```python
from build123d import *

# Parameters (mm, degrees)
SKETCH1_W               = 249.6
SKETCH1_H               = 340.9
SKETCH1_R               = 2.1
SKETCH1_R_2             = 2.5
SKETCH1_R_3             = 1.59
SKETCH1_R_4             = 12.5
SKETCH1_W_2             = 33
SKETCH1_H_2             = 90
BOSS_EXTRUDE1_DEPTH     = 5
CUT_EXTRUDE3_DEPTH      = 193
CUT_EXTRUDE3_DEPTH_BACK = 193
CUT_EXTRUDE6_DEPTH      = 6
SKETCH8_R               = 2
SKETCH8_R_2             = 2.1
SKETCH8_R_3             = 2.058578644
SKETCH8_R_4             = 4
SKETCH8_R_5             = 4.3
CUT_EXTRUDE7_DEPTH      = 6
SKETCH9_R               = 12.5
SKETCH9_R_2             = 2.1
CUT_EXTRUDE8_DEPTH      = 6


with BuildPart() as part:
    # Sketch1 → Boss-Extrude1 (new body)
    with BuildSketch(Plane.XY):
        with Locations((124.8, -170.45)):
            Rectangle(SKETCH1_W, SKETCH1_H)
        with Locations((104.3, -14)):
            Circle(SKETCH1_R, mode=Mode.SUBTRACT)
        with Locations((245.6, -26.5)):
            Circle(SKETCH1_R_2, mode=Mode.SUBTRACT)
        with Locations((245.6, -77.5)):
            Circle(SKETCH1_R_2, mode=Mode.SUBTRACT)
        with Locations((145.3, -14)):
            Circle(SKETCH1_R, mode=Mode.SUBTRACT)
        with Locations((179.16, -36.375)):
            Circle(SKETCH1_R_3, mode=Mode.SUBTRACT)
        with Locations((179.16, -67.625)):
            Circle(SKETCH1_R_3, mode=Mode.SUBTRACT)
        with Locations((124.8, -14)):
            Circle(SKETCH1_R_4, mode=Mode.SUBTRACT)
        with Locations((141.06, -36.375)):
            Circle(SKETCH1_R_3, mode=Mode.SUBTRACT)
        with Locations((153.76, -36.375)):
            Circle(SKETCH1_R_3, mode=Mode.SUBTRACT)
        with Locations((166.46, -36.375)):
            Circle(SKETCH1_R_3, mode=Mode.SUBTRACT)
        with Locations((141.06, -67.625)):
            Circle(SKETCH1_R_3, mode=Mode.SUBTRACT)
        with Locations((153.76, -67.625)):
            Circle(SKETCH1_R_3, mode=Mode.SUBTRACT)
        with Locations((166.46, -67.625)):
            Circle(SKETCH1_R_3, mode=Mode.SUBTRACT)
        with Locations((83.14, -67.625)):
            Circle(SKETCH1_R_3, mode=Mode.SUBTRACT)
        with Locations((95.84, -67.625)):
            Circle(SKETCH1_R_3, mode=Mode.SUBTRACT)
        with Locations((108.54, -67.625)):
            Circle(SKETCH1_R_3, mode=Mode.SUBTRACT)
        with Locations((83.14, -36.375)):
            Circle(SKETCH1_R_3, mode=Mode.SUBTRACT)
        with Locations((95.84, -36.375)):
            Circle(SKETCH1_R_3, mode=Mode.SUBTRACT)
        with Locations((108.54, -36.375)):
            Circle(SKETCH1_R_3, mode=Mode.SUBTRACT)
        with Locations((70.44, -67.625)):
            Circle(SKETCH1_R_3, mode=Mode.SUBTRACT)
        with Locations((70.44, -36.375)):
            Circle(SKETCH1_R_3, mode=Mode.SUBTRACT)
        with Locations((4, -77.5)):
            Circle(SKETCH1_R_2, mode=Mode.SUBTRACT)
        with Locations((4, -26.5)):
            Circle(SKETCH1_R_2, mode=Mode.SUBTRACT)
        with Locations((201.66, -52)):
            Rectangle(SKETCH1_W_2, SKETCH1_H_2, mode=Mode.SUBTRACT)
        with BuildLine():
            Line((145.8225, -36.375), (145.8225, -41.375))
            ThreePointArc((145.8225, -41.375), (147.41, -42.9625), (148.9975, -41.375))
            Line((148.9975, -41.375), (148.9975, -36.375))
            ThreePointArc((148.9975, -36.375), (147.41, -34.7875), (145.8225, -36.375))
        make_face(mode=Mode.SUBTRACT)
        with BuildLine():
            Line((158.52, -36.375), (158.52, -41.375))
            ThreePointArc((158.52, -41.375), (160.11, -42.965), (161.7, -41.375))
            Line((161.7, -41.375), (161.7, -36.375))
            ThreePointArc((161.7, -36.375), (160.11, -34.785), (158.52, -36.375))
        make_face(mode=Mode.SUBTRACT)
        with BuildLine():
            Line((171.22, -36.375), (171.22, -41.375))
            ThreePointArc((171.22, -41.375), (172.81, -42.965), (174.4, -41.375))
            Line((174.4, -41.375), (174.4, -36.375))
            ThreePointArc((174.4, -36.375), (172.81, -34.785), (171.22, -36.375))
        make_face(mode=Mode.SUBTRACT)
        with BuildLine():
            Line((145.8225, -67.625), (145.8225, -72.625))
            ThreePointArc((145.8225, -72.625), (147.41, -74.2125), (148.9975, -72.625))
            Line((148.9975, -72.625), (148.9975, -67.625))
            ThreePointArc((148.9975, -67.625), (147.41, -66.0375), (145.8225, -67.625))
        make_face(mode=Mode.SUBTRACT)
        with BuildLine():
            Line((158.52, -67.625), (158.52, -72.625))
            ThreePointArc((158.52, -72.625), (160.11, -74.215), (161.7, -72.625))
            Line((161.7, -72.625), (161.7, -67.625))
            ThreePointArc((161.7, -67.625), (160.11, -66.035), (158.52, -67.625))
        make_face(mode=Mode.SUBTRACT)
        with BuildLine():
            Line((171.22, -67.625), (171.22, -72.625))
            ThreePointArc((171.22, -72.625), (172.81, -74.215), (174.4, -72.625))
            Line((174.4, -72.625), (174.4, -67.625))
            ThreePointArc((174.4, -67.625), (172.81, -66.035), (171.22, -67.625))
        make_face(mode=Mode.SUBTRACT)
        with BuildLine():
            Line((103.7775, -36.375), (103.7775, -41.375))
            ThreePointArc((103.7775, -41.375), (102.19, -42.9625), (100.6025, -41.375))
            Line((100.6025, -41.375), (100.6025, -36.375))
            ThreePointArc((100.6025, -36.375), (102.19, -34.7875), (103.7775, -36.375))
        make_face(mode=Mode.SUBTRACT)
        with BuildLine():
            Line((91.08, -36.375), (91.08, -41.375))
            ThreePointArc((91.08, -41.375), (89.49, -42.965), (87.9, -41.375))
            Line((87.9, -41.375), (87.9, -36.375))
            ThreePointArc((87.9, -36.375), (89.49, -34.785), (91.08, -36.375))
        make_face(mode=Mode.SUBTRACT)
        with BuildLine():
            Line((78.38, -36.375), (78.38, -41.375))
            ThreePointArc((78.38, -41.375), (76.79, -42.965), (75.2, -41.375))
            Line((75.2, -41.375), (75.2, -36.375))
            ThreePointArc((75.2, -36.375), (76.79, -34.785), (78.38, -36.375))
        make_face(mode=Mode.SUBTRACT)
        with BuildLine():
            Line((103.7775, -67.625), (103.7775, -72.625))
            ThreePointArc((103.7775, -72.625), (102.19, -74.2125), (100.6025, -72.625))
            Line((100.6025, -72.625), (100.6025, -67.625))
            ThreePointArc((100.6025, -67.625), (102.19, -66.0375), (103.7775, -67.625))
        make_face(mode=Mode.SUBTRACT)
        with BuildLine():
            Line((91.08, -67.625), (91.08, -72.625))
            ThreePointArc((91.08, -72.625), (89.49, -74.215), (87.9, -72.625))
            Line((87.9, -72.625), (87.9, -67.625))
            ThreePointArc((87.9, -67.625), (89.49, -66.035), (91.08, -67.625))
        make_face(mode=Mode.SUBTRACT)
        with BuildLine():
            Line((78.38, -67.625), (78.38, -72.625))
            ThreePointArc((78.38, -72.625), (76.79, -74.215), (75.2, -72.625))
            Line((75.2, -72.625), (75.2, -67.625))
            ThreePointArc((75.2, -67.625), (76.79, -66.035), (78.38, -67.625))
        make_face(mode=Mode.SUBTRACT)
        with Locations((47.94, -52)):
            Rectangle(SKETCH1_W_2, SKETCH1_H_2, mode=Mode.SUBTRACT)
    extrude(amount=BOSS_EXTRUDE1_DEPTH)

    # Sketch4 → Cut-Extrude3 (cut, two sides)
    with BuildSketch(Plane.XY.offset(5)) as cut_extrude3_sk:
        with BuildLine():
            Line((249.6, -161.594545719), (249.6, -280.754609783))
            ThreePointArc((249.6, -280.754609783), (205.980407386, -221.174577751), (249.6, -161.594545719))
        make_face()
    extrude(amount=CUT_EXTRUDE3_DEPTH, mode=Mode.SUBTRACT)
    extrude(cut_extrude3_sk.sketch, amount=-CUT_EXTRUDE3_DEPTH_BACK, mode=Mode.SUBTRACT)

    # Sketch7 → Cut-Extrude6 (cut, through all)
    with BuildSketch(Plane.XY.offset(5)):
        Polygon((249.6, -158.447518206), (126.382609779, -197.494065264), (226.608591706, -274.129323659), (0, -274.129323659), (0, -340.9), (249.6, -340.9), align=None)
    extrude(amount=-CUT_EXTRUDE6_DEPTH, mode=Mode.SUBTRACT)

    # Sketch8 → Cut-Extrude7 (cut, through all)
    with BuildSketch(Plane.XY.offset(5)):
        with Locations((3.008996966, -144.071505353)):
            Circle(SKETCH8_R)
        with Locations((18.194231921, -124.211781303)):
            Circle(SKETCH8_R_2)
        with Locations((22.868721016, -159.256740308)):
            Circle(SKETCH8_R_2)
        with Locations((36.770527851, -169.886404777)):
            Circle(SKETCH8_R_3)
        with Locations((40.391200519, -156.919495761)):
            Circle(SKETCH8_R_4)
        with Locations((38.053955971, -139.397016258)):
            Circle(SKETCH8_R)
        with Locations((20.531476469, -141.734260806)):
            Circle(SKETCH8_R_5)
        with Locations((51.955762806, -150.026680727)):
            Circle(SKETCH8_R_3)
    extrude(amount=-CUT_EXTRUDE7_DEPTH, mode=Mode.SUBTRACT)

    # Sketch9 → Cut-Extrude8 (cut, through all)
    with BuildSketch(Plane.XY.offset(5)):
        with Locations((62.4, -249.129323659)):
            Circle(SKETCH9_R)
        with Locations((82.9, -249.129323659)):
            Circle(SKETCH9_R_2)
        with Locations((41.9, -249.129323659)):
            Circle(SKETCH9_R_2)
        with Locations((207.7, -249.129323659)):
            Circle(SKETCH9_R_2)
        with Locations((166.7, -249.129323659)):
            Circle(SKETCH9_R_2)
        with Locations((187.2, -249.129323659)):
            Circle(SKETCH9_R)
    extrude(amount=-CUT_EXTRUDE8_DEPTH, mode=Mode.SUBTRACT)


solid = part.part
```
Could you check a few things on this model? Use its own coordinates, in mm. A direction names the side the tool comes from. Coordinates: 2 decimals unless noted, no trailing zeros. Loops run counter-clockwise (first coordinate to the right, second up) from the corner with the lowest first, then second, coordinate; pieces in that order, holes last. Notation, with made-up numbers: M 38,-21 L 42,-21 A25 ccw 42,11 Z; hole C 6.25,62.25 d9. An arc over 180 degrees is marked long. Put each result on its own line as item: value. Start each with the question number.
(1) Suppose I cut it at B-B on z = 1.4. Count the separate pieces of the cut face and the enclosed holes in it, then the cut area to 3 significant figures.
(2) I need wall thicknesses on line 1 (X direction, y = -44, z = 4.25); line 2 (Y direction, x = 108.54, z = 2.3) (3 decimals); line 3 (Y direction, x = 159, z = 4.8). Which ranges of each line are inside material? Lowest first, please. Write a range as from..to.
(3) Suppose I cut it at A-A on y = -84.5. Please give me the cut outline in (x, z).
(4) Thinking about a two-plate mould opening in Y: for faces 1 (the face through (212.64, -263.45, 2.54)), 2 (the face through (152.959, -217.815, 2.535)), 3 (the face through (123, -135, 5)), which applies, pulls with the +Y half, pulls with the -Y half, needs draft (parallel to the pull), parting line crosses it, or undercut?
(5) For faces 4 (the face through (188.85, -177.7, 2.54)), 5 (the face through (179.346, -258.853, 2.535)), which set-ups out of +Z, -Z, +X, -X, +Y, -Y let a thin tool reach every point of the face, with its end or its side?
(6) Suppose I cut it at C-C on y = -184. Please give me the cut outline in (x, z).
(7) Suppose I cut it at D-D on x = 231. Please give me the cut outline in (y, z), then the cut area to 3 significant figures.
Solutions:
1. separate pieces: 1
1. enclosed holes: 49
1. area: 52,400 mm2
2. line 1: x = 0..31.44, 64.44..185.16, 218.16..249.6
2. line 2: y = -274.129..-69.215, -66.035..-37.965, -34.785..0
2. line 3: y = -274.13..-222.43, -187.16..-73.76, -66.49..-42.51, -35.24..0
3. outline: M 0,0 L 31.44,0 L 31.44,5 L 0,5 Z; M 64.44,0 L 185.16,0 L 185.16,5 L 64.44,5 Z; M 218.16,0 L 249.6,0 L 249.6,5 L 218.16,5 Z
4. face 1: undercut
4. face 2: undercut
4. face 3: needs draft
5. face 4: +Z, -Z, +X
5. face 5: +Z, -Z
6. outline: M 0,0 L 168.97,0 L 168.97,5 L 0,5 Z
7. outline: M -164.34,0 L 0,0 L 0,5 L -164.34,5 Z
7. area: 822 mm2
